For this review, take the finished solid that the model builds, in its own axes (mm). A direction names the side the tool comes from. Give positions to 0.01 mm unless a question says otherwise; leave off trailing zeros. Loops run counter-clockwise (first coordinate to the right, second up) from the corner with the lowest first, then second, coordinate; pieces in that order, holes last.
```python
from build123d import *

# Parameters (mm, degrees)
F3_D            = 2.35
F3_COPIES_COUNT = 4
F7_D            = 2.1
F7_DEPTH        = 8.5
F7_START        = 0.0500046
F7_TIP          = 0.63090365


# Not quite as in the source:
# - a pattern or mirror of a feature is missing from the dataset's text; its kind, count and spacing are read off the source's solid


with BuildPart() as f1:
    # F0 (on Front) → F1 (revolve)
    with BuildSketch(Plane.XZ):
        Polygon((-6.35, 4.699), (-6.35, 3), (6.35, 3), (6.35, 4.699), (3.175, 4.699), (3.175, 11.049), (-3.175, 11.049), (-3.175, 4.699), align=None)
    revolve(axis=Axis((0, 0, 0), (1, 0, 0)))

    # F3 (through all)
    with Locations(Plane(origin=(-3.175, 0, 0), x_dir=(0, -1, 0), z_dir=(-1, 0, 0))):
        with Locations((5.6126600757, 5.6126600757)):
            f3 = Hole(F3_D / 2)

    # F3_copies: F3 ×4 about axis
    f3_copies_axis = Axis((0, 0, 0), (1, 0, 0))
    for i in range(1, F3_COPIES_COUNT):
        add(f3.rotate(f3_copies_axis, i * 360 / F3_COPIES_COUNT), mode=Mode.SUBTRACT)

    # F7
    # its depths count from where the whole tool has entered the part; down to there all is cleared
    with Locations(Plane.XY.offset(11.049).offset(-F7_START)):
        with Locations((0, 0)):
            Hole(F7_D / 2, depth=F7_DEPTH)
            with Locations((0, 0, -(F7_DEPTH + F7_TIP / 2))):  # 118° drill point
                Cone(0, F7_D / 2, F7_TIP, mode=Mode.SUBTRACT)


solid = f1.part
```
Item 1: Take a section at B-B on y = 0. Give the boundary of the cut face in (x, z) (3 decimals), and give its area (3 significant figures).
Answer:
outline: (-6.35, -4.699) - (-3.175, -4.699) - (-3.175, -11.049) - (3.175, -11.049) - (3.175, -4.699) - (6.35, -4.699) - (6.35, -3) - (-6.35, -3) - close; (-6.35, 3) - (-1.05, 3) - (-1.05, 11.049) - (-3.175, 11.049) - (-3.175, 4.699) - (-6.35, 4.699) - close; (1.05, 3) - (6.35, 3) - (6.35, 4.699) - (3.175, 4.699) - (3.175, 11.049) - (1.05, 11.049) - close
area: 107 mm2
Item 2: Take a section at C-C on z = 5. Give the boundary of the cut face in (x, y) (3 decimals).
Answer:
outline: (-3.175, -9.853) - (3.175, -9.853) - (3.175, -6.615) - (-3.175, -6.615) - close; (-3.175, -4.61) - (3.175, -4.61) - (3.175, 4.61) - (-3.175, 4.61) - close; (-3.175, 6.615) - (3.175, 6.615) - (3.175, 9.853) - (-3.175, 9.853) - close; hole circle Ø2.1 at (0, 0)
Item 3: Clearance check with flat-ended pins moving along their axes: pin 1 Ø2 at (y, z) = (5.61, -5.61) entering from +X; pin 2 Ø1 at (x, y) = (0, -3.5) entering from -Z; pin 3 Ø9.5 at (y, z) = (0, 0) entering from -X; pin 4 Ø2.5 at (y, z) = (-5.61, -5.61) entering from -X (3 decimals). State where each tip first meets the part, or that it passes through.
Answer:
pin 1: passes through
pin 2: stops at z = -10.63
pin 3: stops at x = -6.35
pin 4: stops at x = -3.175
Item 4: Take a section at D-D on x = 0.5. Give the boundary of the cut face in (y, z) (3 decimals).
Answer:
outline: (-0.923, 2.854) - (-0.923, 11.01) arc R11.049 ccw (long way) to (0.923, 11.01) - (0.923, 2.854) arc R3 cw (long way) to start; hole circle Ø2.35 at (-5.613, -5.613); hole circle Ø2.35 at (-5.613, 5.613); hole circle Ø2.35 at (5.613, -5.613); hole circle Ø2.35 at (5.613, 5.613)
Item 5: For L1, parallel to Y at x = -2.5, z = 0; L2, parallel to X at y = 0.25, z = 8.75 (3 decimals); L3, parallel to X at y = -4, z = -9.5 (3 decimals), list the stretches that pass through material, from the lowest coordinate up.
Answer:
L1: y = -11.05 to -3, 3 to 11.05
L2: x = -3.175 to -1.02, 1.02 to 3.175
L3: x = -3.175 to 3.175
Item 6: Tool access review of faces 1 (the cylindrical face through (4.74, -4.66, -0.61)), 2 (the flat face through (-3.175, 5, 0)), 3 (the cylindrical face through (-1, 0.32, 6.87)): name each direction out of +Z, -Z, +X, -X, +Y, -Y from which nothing blocks a thin tool from reaching the whole face with its end or side.
Answer:
face 1: +X
face 2: -X
face 3: +Z
Item 7: The part is to be moulded in two halves that separate along Z. For faces 4 (the flat face through (-6.35, 1, 3)), 5 (the cylindrical face through (0.1, 1.8, -2.4)), 6 (the cylindrical face through (-0.044, -10.955, -1.438)), say which applies: released by +Z, released by -Z, zero draft, split by the parting line, or undercut.
Answer:
face 4: zero draft
face 5: undercut
face 6: split by the parting line
Item 8: Take a section at A-A on z = 0. Give the boundary of the cut face in (x, y) (3 decimals), and give its area (3 significant figures).
Answer:
outline: (-6.35, -4.699) - (-3.175, -4.699) - (-3.175, -11.049) - (3.175, -11.049) - (3.175, -4.699) - (6.35, -4.699) - (6.35, -3) - (-6.35, -3) - close; (-6.35, 3) - (6.35, 3) - (6.35, 4.699) - (3.175, 4.699) - (3.175, 11.049) - (-3.175, 11.049) - (-3.175, 4.699) - (-6.35, 4.699) - close
area: 124 mm2
